Here's how the part is built. I have some questions about the finished solid (model axes, mm). A direction names the side the tool comes from. Round coordinates to 2 decimals unless told otherwise and drop trailing zeros. Loops run counter-clockwise (first coordinate to the right, second up) from the corner with the lowest first, then second, coordinate; pieces in that order, holes last. Notation, with made-up numbers: M -8.5,15 L 12.5,15 A23 cw 12.5,23 Z; hole C -5.75,10.5 d9. An arc over 180 degrees is marked long. Answer as a JSON object with one key per item and string values.
from build123d import *

# Parameters (mm, degrees)
CUT_EXTRUDE1_DEPTH = 1.27


with BuildPart() as part:
    # Sketch1 → Revolve1 (revolve)
    with BuildSketch(Plane.XY):
        with BuildLine():
            Line((-2, 0), (-3.8, 0))
            ThreePointArc((-3.8, 0), (-3.038270032, 1.319559026), (-1.79477003, 2.2))
            Line((-1.79477003, 2.2), (0, 2.2))
            Line((0, 2.2), (0, -14))
            Line((0, -14), (-2, -14))
            Line((-2, -14), (-2, 0))
        make_face()
    revolve(axis=Axis((0, -14, 0), (0, 1, 0)))

    # Sketch2 → Cut-Extrude1 (cut)
    with BuildSketch(Plane(origin=(0, 2.2, 0), x_dir=(1, 0, 0), z_dir=(0, 1, 0))):
        Polygon((-1.25, 0.721687836), (-1.25, -0.721687836), (0, -1.443375673), (1.25, -0.721687836), (1.25, 0.721687836), (0, 1.443375673), align=None)
    extrude(amount=-CUT_EXTRUDE1_DEPTH, mode=Mode.SUBTRACT)


solid = part.part
Item 1: On a 3-axis mill with a long thin cutter (end or side, diameter ignored), from which of +Z, -Z, +X, -X, +Y, -Y can I reach the whole of each face in a straight line? I mean faces 1 (the face through (0.63, 1.57, -1.08)), 2 (the face through (2, 0, -2)), 3 (the face through (0, -14, 0)). Say none if no direction works.
Resolved:
{"face 1": "+Y", "face 2": "-Y", "face 3": "+Z, -Z, +X, -X, -Y"}
Item 2: I'm going to push flat-ended pins straight in: pin 1 Ø3 at (y, z) = (-11.5, 1.5) entering from -X; pin 2 Ø2 at (y, z) = (-4, 0.5) entering from +X; pin 3 Ø3 at (x, z) = (-3, 2.5) entering from +Y. Where does each tip first touch, or does it pass through?
Resolved:
{"pin 1": "x = -2", "pin 2": "x = 2", "pin 3": "y = 1.87"}
Item 3: I want a section at A-A, the plane y = -1.25. Please give me the cut outline in (x, z).
Resolved:
{"outline": "C 0,0 d4"}
Item 4: Please list where these lines run through material, in increasing order: probe 1 along Y at (x, z) = (1, 0.5); probe 2 along Z at (x, y) = (0, -11.5); probe 3 along Y at (x, z) = (1.75, -1.5). Write a range as from..to.
Resolved:
{"probe 1": "-14..0.93", "probe 2": "-2..2", "probe 3": "0..1.93"}
